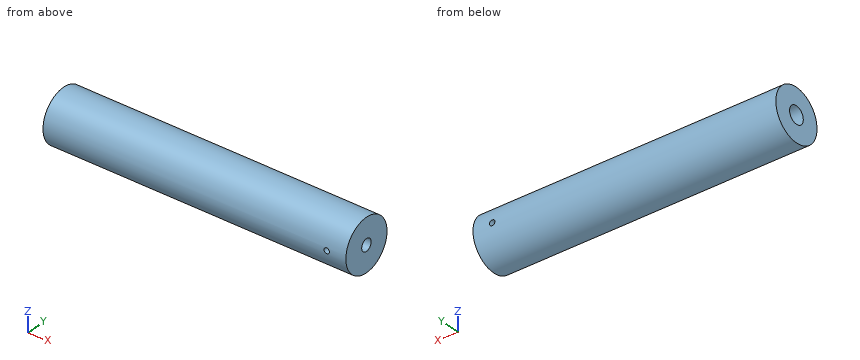
```python
from build123d import *

# Parameters (mm, degrees)
SKETCH1_R               = 12
BOSS_EXTRUDE1_DEPTH     = 140
CUT_EXTRUDE1_DEPTH      = 120
CUT_EXTRUDE1_DEPTH_BACK = 120
SKETCH2_R               = 1.25
SKETCH3_R               = 2.75
CUT_EXTRUDE2_DEPTH      = 42
SKETCH4_R               = 4
CUT_EXTRUDE3_DEPTH      = 70


with BuildPart() as part:
    # Sketch1 → Boss-Extrude1 (new body)
    with BuildSketch(Plane(origin=(0, 0, 0), x_dir=(0, 0, -1), z_dir=(1, 0, 0))):
        Circle(SKETCH1_R)
    extrude(amount=BOSS_EXTRUDE1_DEPTH)

    # Sketch2 → Cut-Extrude1 (cut, two sides: drawn at the far end of the back side and taken through both)
    with BuildSketch(Plane(origin=(0, 0, 0), x_dir=(1, 0, 0), z_dir=(0, 1, 0)).offset(-CUT_EXTRUDE1_DEPTH_BACK)):
        with Locations(Location((131.130079525, 0, 0), (0, 0, 270))):
            Circle(SKETCH2_R)
    extrude(amount=CUT_EXTRUDE1_DEPTH + CUT_EXTRUDE1_DEPTH_BACK, mode=Mode.SUBTRACT)

    # Sketch3 → Cut-Extrude2 (cut)
    with BuildSketch(Plane(origin=(140, 0, 0), x_dir=(0, 0, -1), z_dir=(1, 0, 0))):
        Circle(SKETCH3_R)
    extrude(amount=-CUT_EXTRUDE2_DEPTH, mode=Mode.SUBTRACT)

    # Sketch4 → Cut-Extrude3 (cut)
    with BuildSketch(Plane.ZY):
        Circle(SKETCH4_R)
    extrude(amount=-CUT_EXTRUDE3_DEPTH, mode=Mode.SUBTRACT)


solid = part.part
```
Geometry check sheet. Reference: the model listing, model coordinates, mm. Round coordinates to 2 decimals unless told otherwise and drop trailing zeros. Loops run counter-clockwise (first coordinate to the right, second up) from the corner with the lowest first, then second, coordinate; pieces in that order, holes last. Notation, with made-up numbers: M 57.5,23 L 93.5,23 A27 ccw 93.5,50 Z; hole C 50.25,-22 d11. An arc over 180 degrees is marked long. Return JSON: item names as keys, results as strings. Group by question number.
(1) Section check D-D, the plane y = 7.5. Enter the section's corners in (x, z), and give its area (3 significant figures).
(2) Section check A-A, the plane z = 0. Enter the section's corners in (x, y).
(3) Section check B-B, the plane y = 0. Enter the section's corners in (x, z), and give its area (3 significant figures).
(4) Scan lines: line 1 along Y through (x, z) = (117.5, 0); line 2 along Y through (x, z) = (52, 0); line 3 along X through (y, z) = (-4.25, 0). Record each from-to range of solid material in increasing order. Write a range as [from, to].
(5) Section check C-C, the plane x = 66. Enter the section's corners in (y, z), and give its area (3 significant figures).
(6) Go/stop test with flat-tipped pins: pin 1 (1.5 mm diameter, centred on x = 117.5, z = 6.5, fed in from +Y); pin 2 (1.5 mm diameter, centred on x = 55, z = -4.5, fed in from +Y); pin 3 (2.5 mm diameter, centred on y = 1.5, z = -0.5, fed in from -X). Record where each tip stops, or that it passes through.
Data:
{
 "1": {"outline": "M 0,-9.37 L 140,-9.37 L 140,9.37 L 0,9.37 Z; hole C 131.13,0 d2.5", "area": "2,620 mm²"},
 "2": {"outline": "M 0,-12 L 129.88,-12 L 129.88,-2.75 L 98,-2.75 L 98,2.75 L 129.88,2.75 L 129.88,12 L 0,12 L 0,4 L 70,4 L 70,-4 L 0,-4 Z; M 132.38,-12 L 140,-12 L 140,-2.75 L 132.38,-2.75 Z; M 132.38,2.75 L 140,2.75 L 140,12 L 132.38,12 Z"},
 "3": {"outline": "M 0,-12 L 140,-12 L 140,-2.75 L 98,-2.75 L 98,2.75 L 140,2.75 L 140,12 L 0,12 L 0,4 L 70,4 L 70,-4 L 0,-4 Z", "area": "2,570 mm²"},
 "4": {"line 1": "[-12, -2.75], [2.75, 12]", "line 2": "[-12, -4], [4, 12]", "line 3": "[0, 129.88], [132.38, 140]"},
 "5": {"outline": "C 0,0 d24; hole C 0,0 d8", "area": "402 mm²"},
 "6": {"pin 1": "y = 10.53", "pin 2": "y = 11.4", "pin 3": "x = 70"}
}
